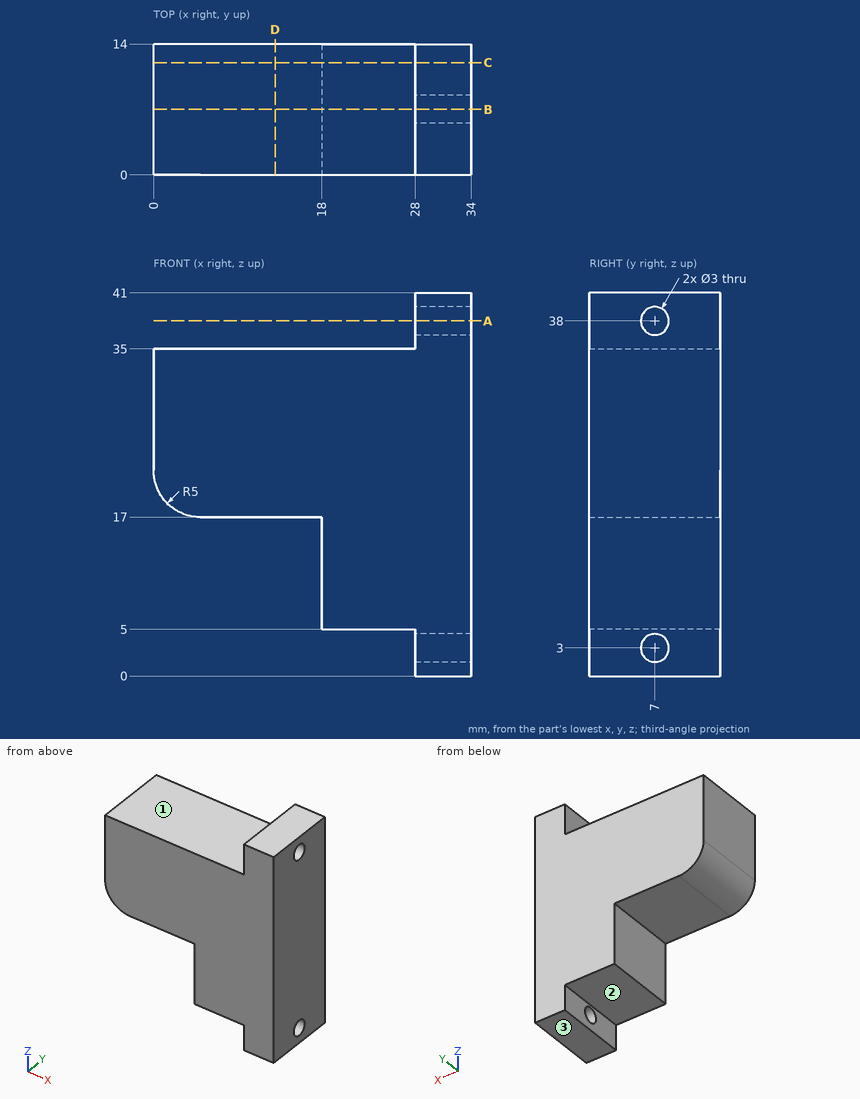
Check sheet for the drawn part. Datum: minimum x, y, z corner. Units: mm. A direction names the side the tool comes from. Give positions to 0.01 mm unless a question says otherwise; leave off trailing zeros. Write each loop counter-clockwise with the first axis right and the second up, starting at its lowest first coordinate (ties: lowest second). Pieces come first, ordered by that corner, then holes. Notation, with made-up numbers: M 6,20.5 L 53,20.5 A16 cw 53,49.5 Z; hole C -8.5,66.25 d6. An arc over 180 degrees is marked long. Write item = value, one per line.
(1) Access from +Z, -Z, +X, -X, +Y, -Y to the whole of each face (thin tool, end or side, straight path). Record for the marked faces 1, 2 and 3.
Found:
face_1 = +Z, -X, +Y, -Y
face_2 = -Z, -X, +Y, -Y
face_3 = -Z, +X, -X, +Y, -Y
(2) Go/stop test with flat-tipped pins: pin 1 Ø5 at (y, z) = (7, 3) entering from -X; pin 2 Ø5.5 at (y, z) = (5.5, 1.5) entering from -X; pin 3 Ø6.5 at (x, y) = (12, 9) entering from -Z. Record where each tip stops, or that it passes through.
Found:
pin_1 = 18
pin_2 = 28
pin_3 = 17
(3) Sectioned sample at B-B (y = 7). Record the cut outline in (x, z).
Found:
outline = M 0,22 A5 ccw 5,17 L 18,17 L 18,5 L 28,5 L 28,4.5 L 34,4.5 L 34,36.5 L 28,36.5 L 28,35 L 0,35 Z; M 28,0 L 34,0 L 34,1.5 L 28,1.5 Z; M 28,39.5 L 34,39.5 L 34,41 L 28,41 Z
(4) Sectioned sample at C-C (y = 12). Record the cut outline in (x, z), then the cut area to 3 significant figures.
Found:
outline = M 0,22 A5 ccw 5,17 L 18,17 L 18,5 L 28,5 L 28,0 L 34,0 L 34,41 L 28,41 L 28,35 L 0,35 Z
area = 865 mm2
(5) Material ranges on line 1 (Y direction, x = 30, z = 3); line 2 (X direction, y = 6.5, z = 6.5); line 3 (Z direction, x = 15, y = 4.75), recorded low to high.
Found:
line_1 = 0 to 5.5, 8.5 to 14
line_2 = 18 to 34
line_3 = 17 to 35
(6) Sectioned sample at D-D (x = 13). Record the cut outline in (y, z), then the cut area to 3 significant figures.
Found:
outline = M 0,17 L 14,17 L 14,35 L 0,35 Z
area = 252 mm2
(7) Sectioned sample at A-A (z = 38). Record the cut outline in (x, y).
Found:
outline = M 28,0 L 34,0 L 34,5.5 L 28,5.5 Z; M 28,8.5 L 34,8.5 L 34,14 L 28,14 Z
